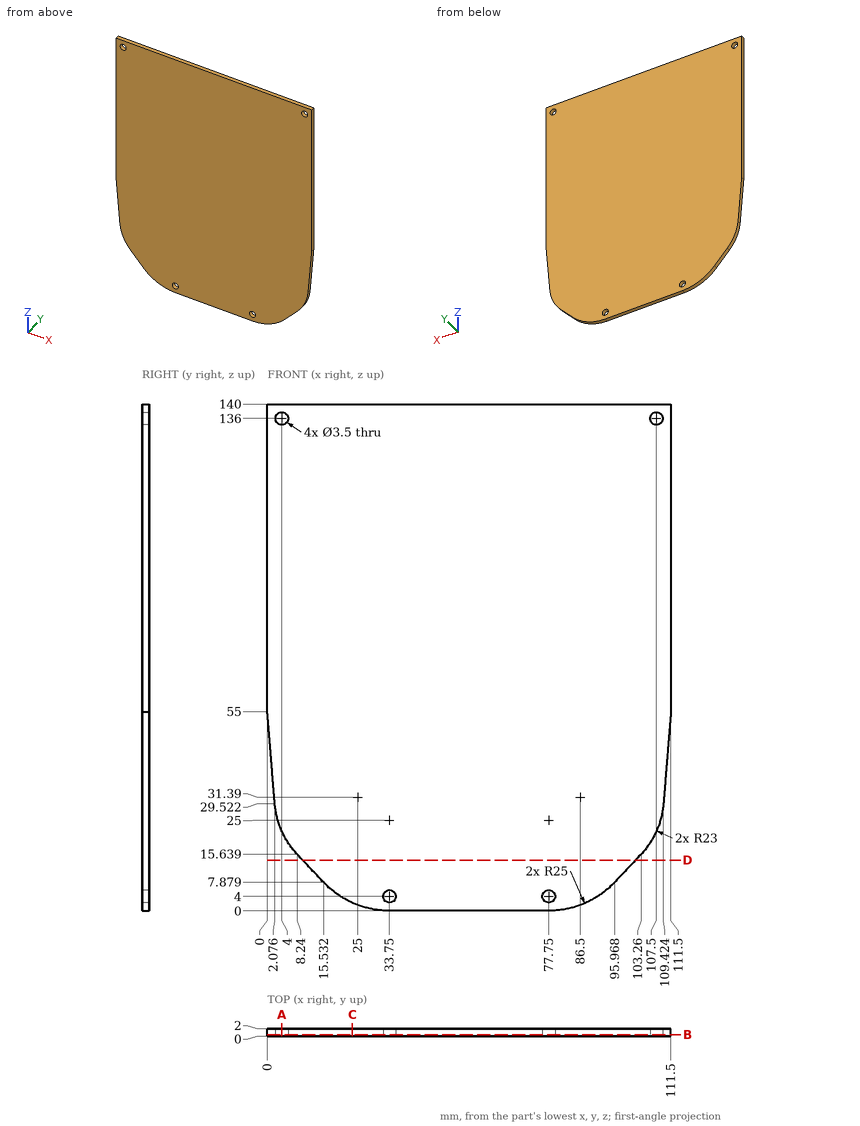
Answer from the drawing. Dimensions are ordinates in mm from the lowest x, y and z of the part. Give positions to 0.01 mm unless a question says otherwise; leave off trailing zeros. Write each loop counter-clockwise with the first axis right and the second up, starting at its lowest first coordinate (ties: lowest second). Pieces come first, ordered by that corner, then holes. Notation, with made-up numbers: (28, -37) -> (36, -37) arc R29 ccw to (36, 0) -> close; hole circle Ø11 at (-18.5, -18). An arc over 180 degrees is marked (long way). Use a Markdown table: item, result.
(1) Section B-B, the plane y = 0.4 is taken. Determine the outline of the cut face in (x, z).
Return value:
| item | result |
|---|---|
| outline | (0, 55) -> (2.08, 29.52) arc R23 ccw to (8.24, 15.64) -> (15.53, 7.88) arc R25 ccw to (33.75, 0) -> (77.75, 0) arc R25 ccw to (95.97, 7.88) -> (103.26, 15.64) arc R23 ccw to (109.42, 29.52) -> (111.5, 55) -> (111.5, 140) -> (0, 140) -> close; hole circle Ø3.5 at (4, 136); hole circle Ø3.5 at (33.75, 4); hole circle Ø3.5 at (77.75, 4); hole circle Ø3.5 at (107.5, 136) |
(2) A flat-ended cylindrical pin translates along its axis: P1, Ø2, axis at x = 33.75, z = 4, coming from the +Y side. Find the tip coordinate at first contact, or state that the pin passes through.
Return value:
| item | result |
|---|---|
| P1 | through |
(3) Find the intervals of material crossed by probe 1 along X at (y, z) = (1.1, 136); probe 2 along Z at (x, y) = (77.75, 0.7); probe 3 along Z at (x, y) = (79, 1) (1 decimal), in increasing order. Write a range as from..to.
Return value:
| item | result |
|---|---|
| probe 1 | 0..2.25, 5.75..105.75, 109.25..111.5 |
| probe 2 | 0..2.25, 5.75..140 |
| probe 3 | 0..2.8, 5.2..140 |
(4) Section D-D, the plane z = 14 is taken. Determine the outline of the cut face in (x, y).
Return value:
| item | result |
|---|---|
| outline | (9.78, 0) -> (101.72, 0) -> (101.72, 2) -> (9.78, 2) -> close |
(5) Section A-A, the plane x = 4 is taken. Determine the outline of the cut face in (y, z), then the cut area to 3 significant figures.
Return value:
| item | result |
|---|---|
| outline | (0, 22.01) -> (2, 22.01) -> (2, 134.25) -> (0, 134.25) -> close; (0, 137.75) -> (2, 137.75) -> (2, 140) -> (0, 140) -> close |
| area | 229 mm2 |
(6) Section C-C, the plane x = 23.5 is taken. Determine the outline of the cut face in (y, z).
Return value:
| item | result |
|---|---|
| outline | (0, 2.2) -> (2, 2.2) -> (2, 140) -> (0, 140) -> close |
